```python
from build123d import *

# Parameters (mm, degrees)
F1_DEPTH = 101.6
F2_DEPTH = 25.4
F3_R     = 12.7
F4_DEPTH = 127.001
F5_R     = 12.7
F6_DEPTH = 25.401


with BuildPart() as f1:
    # F0 (on Top) → F1 (new body)
    with BuildSketch(Plane.XY):
        Polygon((63.1043637723, -63.0199108629), (63.1043637723, -39.3234714866), (-38.4956362277, -39.3234714866), (-38.4956362277, -63.0199108629), (38.0817614496, -63.0199108629), align=None)
    extrude(amount=F1_DEPTH)

    # F0 (on Top) → F2 (join)
    with BuildSketch(Plane.XY):
        Polygon((63.1043637723, 63.9800891371), (-13.0956362277, 63.9800891371), (-13.0956362277, 13.1800891371), (-38.4956362277, 13.1800891371), (-38.4956362277, -39.3234714866), (63.1043637723, -39.3234714866), align=None)
    extrude(amount=F2_DEPTH)

    # F3 (on face) → F4 (cut, through all)
    with BuildSketch(Plane.XZ.offset(63.0199108629)):
        with Locations((0, 76.2)):
            Circle(F3_R)
    extrude(amount=-F4_DEPTH, mode=Mode.SUBTRACT)

    # F5 (on face) → F6 (cut, through all)
    with BuildSketch(Plane.XY.offset(25.4)):
        with Locations((25.0043637723, 38.5800891371)):
            Circle(F5_R)
    extrude(amount=-F6_DEPTH, mode=Mode.SUBTRACT)


solid = f1.part
```
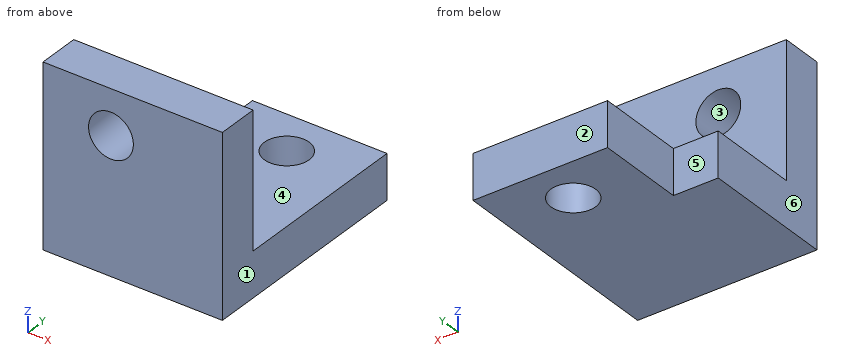
For this review, take the finished solid that the model builds, in its own axes (mm). Face numbers are marked on the shaded views. A direction names the side the tool comes from. Round coordinates to 2 decimals unless told otherwise and drop trailing zeros. Write each loop counter-clockwise with the first axis right and the second up, starting at its lowest first coordinate (ties: lowest second). Pieces come first, ordered by that corner, then holes. Notation, with made-up numbers: (-1.5, -21.5) -> (40.5, -21.5) arc R24 ccw to (40.5, -7.5) -> close; hole circle Ø1 at (62, 63). An arc over 180 degrees is marked (long way). One line per question, with ' | ' between items. Start each with the question number.
(1) For line 1 along Z through (x, y) = (0, -49); line 2 along X through (y, z) = (-43, 76); line 3 along Y through (x, z) = (-29, 90.5), list the stretches that pass through material, from the lowest coordinate up. Write a range as from..to.
(2) Add section B-B, the plane z = 76.2. Write out the cut boundary in (x, y).
(3) Tool access review of the marked faces 4, 5 and 6: name each direction out of +Z, -Z, +X, -X, +Y, -Y from which nothing blocks a thin tool from reaching the whole face with its end or side.
(4) Add section C-C, the plane y = 43. Write out the cut boundary in (x, z).
(5) Add section A-A, the plane x = 0. Write out the cut boundary in (y, z), plus the area to 3 significant figures.
(6) Add section D-D, the plane z = 9. Write out the cut boundary in (x, y).
(7) Insertion check: P1, Ø7.5, axis at y = 29, z = 18.5, coming from the -X side; P2, Ø8, axis at x = -5.5, z = 66, coming from the +Y side; P3, Ø12.5, axis at x = -23, z = 13.5, coming from the +Y side. Each pin has a flat end and moves straight along its axis. Give the tip position at first contact, or say it passes through.
(8) Mouldability with a two-part tool opening along X and no side actions: class the marked faces 1, 2 and 3 as released by +X, released by -X, zero draft, split by the parting line, or undercut.
Answer list:
1) line 1: 0..63.5, 88.9..101.6 | line 2: -38.5..-12.7, 12.7..63.1 | line 3: -63.02..-39.32
2) outline: (-38.5, -63.02) -> (-12.7, -63.02) -> (-12.7, -39.32) -> (-38.5, -39.32) -> close; (12.7, -63.02) -> (63.1, -63.02) -> (63.1, -39.32) -> (12.7, -39.32) -> close
3) face 4: +Z, +X, -X, +Y | face 5: +Z, -Z, -X, +Y | face 6: +Z, -Z, -X, +Y, -Y
4) outline: (-13.1, 0) -> (13.1, 0) -> (13.1, 25.4) -> (-13.1, 25.4) -> close; (36.91, 0) -> (63.1, 0) -> (63.1, 25.4) -> (36.91, 25.4) -> close
5) outline: (-63.02, 0) -> (63.98, 0) -> (63.98, 25.4) -> (-39.32, 25.4) -> (-39.32, 63.5) -> (-63.02, 63.5) -> close; (-63.02, 88.9) -> (-39.32, 88.9) -> (-39.32, 101.6) -> (-63.02, 101.6) -> close | area: 4,430 mm²
6) outline: (-38.5, -63.02) -> (63.1, -63.02) -> (63.1, 63.98) -> (-13.1, 63.98) -> (-13.1, 13.18) -> (-38.5, 13.18) -> close; hole circle Ø25.4 at (25, 38.58)
7) P1: x = -13.1 | P2: y = -39.32 | P3: y = 13.18
8) face 1: released by +X | face 2: zero draft | face 3: undercut
